Autodesk Inventor part; units mm, degrees
ref_plane "YZ Plane" through (0, 0, 0) normal (1, 0, 0) x (0, 1, 0)
ref_plane "XZ Plane" through (0, 0, 0) normal (0, 1, 0) x (-1, 0, 0)
ref_plane "XY Plane" through (0, 0, 0) normal (0, 0, 1) x (1, 0, 0)
sketch "Sketch1" plane through (0, 0, 0) normal (1, 0, 0) x (0, 1, 0)
  line L0 (0, 0) -> (212.4, 0)
  line L1 (212.4, 0) -> (212.4, -142)
  line L2 (212.4, -142) -> (0, -142)
  line L3 (0, -142) -> (0, 0)
  dimension "d0" = 212.4
  dimension "d1" = 142
extrude "Extrusion1" add sketch "Sketch1" along normal blind 6.5532
sketch "Sketch2" plane through (6.5532, 0, 0) normal (1, 0, 0) x (0, 0, -1)
  line L0 (0, 0) -> (142, 0) construction
  line L1 (48, 32) -> (94, 32) construction
  circle A0 centre (48, 32) radius 4
  circle A1 centre (94, 32) radius 4
  point P0 (71, 0)
  point P1 (71, 32)
  point P2 (71, 0)
  point P3 (71, 0)
  dimension "d9" = 8
  dimension "d10" = 46
  dimension "d11" = 32
extrude "Extrusion2" cut sketch "Sketch2" against normal blind 7.62
sketch "Sketch3" plane through (0, 212.4, 0) normal (0, 1, 0) x (1, 0, 0)
  line L0 (0, 142) -> (0, 0)
  line L1 (0, 0) -> (6.5532, 0)
  line L2 (6.5532, 142) -> (6.5532, 0)
  line L3 (0, 142) -> (6.5532, 142)
  point P0 (0, 0)
extrude "Extrusion3" add sketch "Sketch3" along normal blind 67.056
sketch "Sketch4" plane through (6.5532, 0, 0) normal (1, 0, 0) x (0, 0, -1)
  circle A0 centre (92.7061, 191.9341) radius 3
  circle A1 centre (46.7064, 191.7587) radius 3
  point P0 (0, 0)
extrude "Extrusion4" cut sketch "Sketch4" against normal blind 25.4
properties part number "Z_Gantry_Plate" material "Steel, Mild"
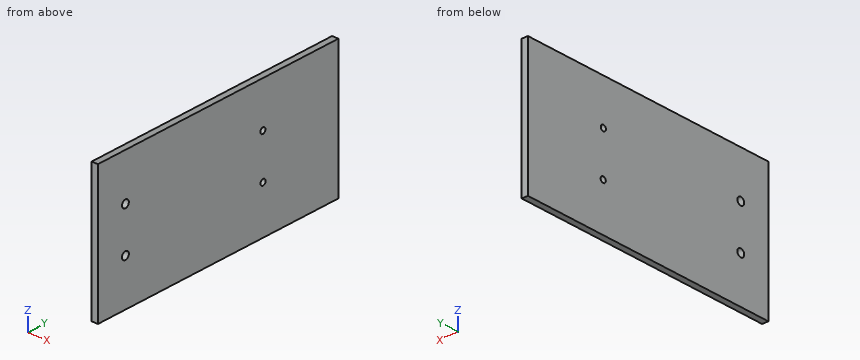
Work out the finished part from the listing and answer in its coordinate system (mm). Coordinates: 2 decimals unless noted, no trailing zeros. Write each loop counter-clockwise with the first axis right and the second up, starting at its lowest first coordinate (ties: lowest second). Pieces come first, ordered by that corner, then holes. Notation, with made-up numbers: M 10.5,12 L 43.5,12 A15 ccw 43.5,29 Z; hole C 72,10 d8. An arc over 180 degrees is marked long. Write item = value, one per line.
1. The part is cut by section A-A (y = 32). Determine the outline of the cut face in (x, z), then the cut area to 3 significant figures.
Solution:
outline = M 0,-142 L 6.55,-142 L 6.55,-98 L 0,-98 Z; M 0,-90 L 6.55,-90 L 6.55,-52 L 0,-52 Z; M 0,-44 L 6.55,-44 L 6.55,0 L 0,0 Z
area = 826 mm2
2. A flat-ended cylindrical pin translates along its axis: pin 1 (7 mm diameter, centred on y = 32, z = -94, fed in from +X). Find the tip coordinate at first contact, or state that the pin passes through.
Solution:
pin_1 = through
3. Straight lines are drawn through the part: line 1 (Y direction, x = 3, z = -45.5); line 2 (Y direction, x = 2.5, z = -94). For each, find the intervals that lie inside material, in ascending order. Write a range as from..to.
Solution:
line_1 = 0..28.88, 35.12..189.01, 194.51..279.46
line_2 = 0..28, 36..189.23, 194.64..279.46
